```python
from build123d import *

# Parameters (mm, degrees)
DODANIE_WYCI_GNI_CIE2_DEPTH     = 80
SZKIC5_W                        = 35.6
SZKIC5_H                        = 35.6
WYTNIJ_WYCI_GNI_CIE1_DEPTH      = 17.8
WYTNIJ_WYCI_GNI_CIE1_DEPTH_BACK = 17.8


with BuildPart() as part:
    # Szkic2 → Dodanie-wyciągnięcie2 (new body)
    with BuildSketch(Plane.XY):
        with BuildLine():
            Line((175.492718802, -24.168338507), (175.492718802, 45.831661493))
            ThreePointArc((175.492718802, 45.831661493), (128.54386121, 39.614419972), (81.570021048, 45.640003906))
            ThreePointArc((81.570021048, 45.640003906), (-1.219530478, 10.831661493), (81.570021048, -23.976680919))
            ThreePointArc((81.570021048, -23.976680919), (128.54386121, -17.951096985), (175.492718802, -24.168338507))
        make_face()
    extrude(amount=DODANIE_WYCI_GNI_CIE2_DEPTH)

    # Szkic5 → Wytnij-wyciągnięcie1 (cut, two sides)
    with BuildSketch(Plane.XY.offset(40)) as wytnij_wyci_gni_cie1_sk:
        with Locations((135.198453221, 10.831661493)):
            Rectangle(SZKIC5_W, SZKIC5_H)
    extrude(amount=WYTNIJ_WYCI_GNI_CIE1_DEPTH, mode=Mode.SUBTRACT)
    extrude(wytnij_wyci_gni_cie1_sk.sketch, amount=-WYTNIJ_WYCI_GNI_CIE1_DEPTH_BACK, mode=Mode.SUBTRACT)


solid = part.part
```
The listing builds one solid part. Answer for the finished solid, in the listing's coordinates (mm). A direction names the side the tool comes from. Give positions to 0.01 mm unless a question says otherwise; leave off trailing zeros. Order: outer loops, then holes, each group sorted by start corner. A loop starts at its lowest first (then second) coordinate and runs counter-clockwise, first axis right, second up. Notation, with made-up numbers: (20.5, 77.5) - (65.5, 77.5) arc R20 cw to (65.5, 95.5) - close; hole circle Ø11 at (46, -12). An arc over 180 degrees is marked (long way). Answer in a Markdown table with one row per item. Add a question column.
Q1. For a pull along X with two mould halves and no side action, classify faces 3 (the flat face through (86, 12, 0)), 4 (the flat face through (175.493, 10, 39)), 5 (the flat face through (135, -6.968, 40)) as released by +X, released by -X, zero draft, split by the parting line, or undercut.
Q2. The part is cut by section D-D (y = 49). Determine the outline of the cut face in (x, z), then the cut area to 3 significant figures.
Q3. Given P1, Ø18, axis at x = 131.5, z = 40.5, coming from the -Y side; P2, Ø18, axis at x = 139, z = 46.5, coming from the +Y side; P3, Ø5, axis at x = 149, z = 29.5, coming from the +Y side, each flat-ended and moving along its own axis, determine where each tip first touches the part or whether it passes through.
Q4. The part is cut by section A-A (y = 19.5). Determine the outline of the cut face in (x, z).
Q5. The part is cut by section C-C (x = 11.5). Determine the outline of the cut face in (y, z), then the cut area to 3 significant figures.
Q6. Which of the six approach directions +Z, -Z, +X, -X, +Y, -Y give full straight-line access (tool end or side, diameter ignored) to faces 1 (the cylindrical face through (129.209, 39.617, 39.44)), 2 (the flat face through (117.398, 11, 40))?
Q7. Find the intervals of material crossed by line 1 along X through (y, z) = (0, 45); line 2 along Z through (x, y) = (151, 26); line 3 along Y through (x, z) = (46.5, 44), in increasing order. Write a range as [from, to].
Q8. The part is cut by section B-B (z = 26). Determine the outline of the cut face in (x, y), then the cut area to 3 significant figures.
Determined:
| question | item | result |
|---|---|---|
| 1 | face 3 | zero draft |
| 1 | face 4 | released by +X |
| 1 | face 5 | undercut |
| 2 | outline | (17.23, 0) - (77.76, 0) - (77.76, 80) - (17.23, 80) - close |
| 2 | area | 4,840 mm² |
| 3 | P1 | stops at y = -18.37 |
| 3 | P2 | stops at y = 40.69 |
| 3 | P3 | stops at y = 41.11 |
| 4 | outline | (-0.44, 0) - (175.49, 0) - (175.49, 80) - (-0.44, 80) - close; hole (117.4, 22.2) - (153, 22.2) - (153, 57.8) - (117.4, 57.8) - close |
| 5 | outline | (-21.99, 0) - (43.66, 0) - (43.66, 80) - (-21.99, 80) - close |
| 5 | area | 5,250 mm² |
| 6 | face 1 | +Z, -Z, +Y |
| 6 | face 2 | none |
| 7 | line 1 | x = [0, 117.4], [153, 175.49] |
| 7 | line 2 | z = [0, 22.2], [57.8, 80] |
| 7 | line 3 | y = [-37.87, 59.53] |
| 8 | outline | (81.57, -23.98) arc R183.2 cw to (175.49, -24.17) - (175.49, 45.83) arc R183.2 cw to (81.57, 45.64) arc R48.71 ccw (long way) to start; hole (117.4, -6.97) - (153, -6.97) - (153, 28.63) - (117.4, 28.63) - close |
| 8 | area | 11,300 mm² |
